Verification items for the finished model (mm, model axes). A direction names the side the tool comes from. Coordinates: 2 decimals unless noted, no trailing zeros. Write each loop counter-clockwise with the first axis right and the second up, starting at its lowest first coordinate (ties: lowest second). Pieces come first, ordered by that corner, then holes. Notation, with made-up numbers: (-38.5, 26.5) -> (7.5, 26.5) arc R22 ccw to (7.5, 58.5) -> close; hole circle Ø5 at (-25, 45.5). An arc over 180 degrees is marked (long way). Use a Markdown table: item, result. Add a question column.
from build123d import *

# Parameters (mm, degrees)
SKETCH1_W           = 37.7
SKETCH1_H           = 32.1
SKETCH1_R           = 2.1
BOSS_EXTRUDE1_DEPTH = 1.5
FILLET1_R           = 3.85


with BuildPart() as part:
    # Sketch1 → Boss-Extrude1 (new body)
    with BuildSketch(Plane(origin=(0, 0, 0), x_dir=(1, 0, 0), z_dir=(0, 1, 0))):
        Rectangle(SKETCH1_W, SKETCH1_H)
        with Locations((15, 11.75)):
            Circle(SKETCH1_R, mode=Mode.SUBTRACT)
        with Locations((15, -11.75)):
            Circle(SKETCH1_R, mode=Mode.SUBTRACT)
        with Locations((-15, 11.75)):
            Circle(SKETCH1_R, mode=Mode.SUBTRACT)
        with Locations((-15, -11.75)):
            Circle(SKETCH1_R, mode=Mode.SUBTRACT)
    extrude(amount=BOSS_EXTRUDE1_DEPTH)

    # Fillet1
    fillet1_edges = [part.edges().sort_by_distance(p)[0] for p in [
        (-18.85, 0.75, -16.05),
        (18.85, 0.75, -16.05),
        (18.85, 0.75, 16.05),
        (-18.85, 0.75, 16.05),
    ]]
    fillet(fillet1_edges, radius=FILLET1_R)

    # Sketch2 → Revolve1 (revolve)
    with BuildSketch(Plane(origin=(0, 0, 0), x_dir=(0, 0, -1), z_dir=(1, 0, 0))):
        Polygon((0, 0), (0, -2.5), (-13.070616019, -2.5), (-16.05, 0), align=None)
    revolve(axis=Axis((0, 0, 0), (0, -1, 0)))


solid = part.part
1) Set-up check for faces 4 (the face through (-16.5, 0, -2.5)), 5 (the face through (14.727, 0.74, -13.832)), 6 (the face through (16.4, 0, -0.1)): record each of +Z, -Z, +X, -X, +Y, -Y from which the full face is reachable in a straight line by a thin tool's end or side.
2) Release check for a two-part mould opening along X. For faces 1 (the face through (-15.273, 0.74, 9.668)), 2 (the face through (0, 1, -16.05)), 3 (the face through (18.85, 1, 0)) record: released by +X, released by -X, zero draft, split by the parting line, or undercut.
3) Thickness scan on L1, parallel to Z at x = -15, y = 0.8; L2, parallel to X at y = 1.2, z = -11.75; L3, parallel to Y at x = -16, z = 3. Record the ranges inside material, lowest first.
4) Cross-section at A-A on y = 0.6. Record the boundary of the cut face in (x, z).
5) Cross-section at B-B on z = -11.75. Give the number of separate pieces and of enclosed holes in the cut face, then the cut area to 3 significant figures.
6) Gauge pin test, flat ends, axial feed: pin 1 (4 mm diameter, centred on x = 15, z = -11.75, fed in from +Y); pin 2 (5.5 mm diameter, centred on x = 15, z = 11.75, fed in from -Y); pin 3 (3 mm diameter, centred on x = 12.5, z = -11, fed in from -Y). Record the tip position at first contact, or that the pin passes through.
Returned:
| question | item | result |
|---|---|---|
| 1 | face 4 | -X, -Y |
| 1 | face 5 | +Y, -Y |
| 1 | face 6 | +X, -Y |
| 2 | face 1 | undercut |
| 2 | face 2 | zero draft |
| 2 | face 3 | released by +X |
| 3 | L1 | z = -16.05 to -13.85, -9.65 to 9.65, 13.85 to 16.05 |
| 3 | L2 | x = -18.85 to -17.1, -12.9 to 12.9, 17.1 to 18.85 |
| 3 | L3 | y = 0 to 1.5 |
| 4 | outline | (-18.85, -12.2) arc R3.85 ccw to (-15, -16.05) -> (15, -16.05) arc R3.85 ccw to (18.85, -12.2) -> (18.85, 12.2) arc R3.85 ccw to (15, 16.05) -> (-15, 16.05) arc R3.85 ccw to (-18.85, 12.2) -> close; hole circle Ø4.2 at (-15, -11.75); hole circle Ø4.2 at (-15, 11.75); hole circle Ø4.2 at (15, -11.75); hole circle Ø4.2 at (15, 11.75) |
| 5 | separate pieces | 3 |
| 5 | enclosed holes | 0 |
| 5 | area | 86.5 mm² |
| 6 | pin 1 | passes through |
| 6 | pin 2 | stops at y = 0 |
| 6 | pin 3 | stops at y = -0.75 |
